Check sheet for the modelled part. Datum: model origin and axes. Units: mm. A direction names the side the tool comes from. Give positions to 0.01 mm unless a question says otherwise; leave off trailing zeros. Order: outer loops, then holes, each group sorted by start corner. A loop starts at its lowest first (then second) coordinate and runs counter-clockwise, first axis right, second up. Notation, with made-up numbers: (78, 17.25) - (103, 17.25) arc R26 cw to (103, 48.25) - close; hole circle Ø1 at (14, 34.25). An arc over 180 degrees is marked (long way). Answer in a Markdown table with one row per item.
from build123d import *

# Parameters (mm, degrees)
SKETCH1_R           = 11
BOSS_EXTRUDE1_DEPTH = 1.5
SKETCH4_R           = 12.5
BOSS_EXTRUDE2_DEPTH = 3
SKETCH5_R           = 1.45
CUT_EXTRUDE1_DEPTH  = 2
SKETCH6_R           = 1.5
CUT_EXTRUDE2_DEPTH  = 2


with BuildPart() as part:
    # Sketch1 → Boss-Extrude1 (new, symmetric)
    with BuildSketch(Plane.XY):
        Circle(SKETCH1_R)
    extrude(amount=BOSS_EXTRUDE1_DEPTH, both=True)

    # Sketch2 → Revolve1 (revolve)
    with BuildSketch(Plane(origin=(0, 0, 0), x_dir=(0, 0, -1), z_dir=(1, 0, 0)), mode=Mode.PRIVATE) as revolve1_sk:
        Polygon((-4.5, 0), (-4.5, 12.5), (-1.5, 11.096489402), (-1.5, 0), align=None)
    revolve(revolve1_sk.sketch.rotate(Axis((0, 0, 0), (0, 0, 1)), 90), axis=Axis((0, 0, 0), (0, 0, 1)))

    # Sketch4 → Boss-Extrude2 (add)
    with BuildSketch(Plane.XY.offset(4.5)):
        Circle(SKETCH4_R)
    extrude(amount=BOSS_EXTRUDE2_DEPTH)

    # Sketch5 → Cut-Extrude1 (cut)
    with BuildSketch(Plane.XY.offset(7.5)):
        with Locations((0, 9.315)):
            Circle(SKETCH5_R)
        with Locations((9.315, 0)):
            Circle(SKETCH5_R)
        with Locations((0, -9.315)):
            Circle(SKETCH5_R)
        with Locations((-9.315, 0)):
            Circle(SKETCH5_R)
    extrude(amount=-CUT_EXTRUDE1_DEPTH, mode=Mode.SUBTRACT)

    # Sketch6 → Cut-Extrude2 (cut)
    with BuildSketch(Plane(origin=(0, 0, -1.5), x_dir=(-1, 0, 0), z_dir=(0, 0, -1))):
        with Locations((0, 7.5)):
            Circle(SKETCH6_R)
        with Locations((7.5, 0)):
            Circle(SKETCH6_R)
        with Locations((0, -7.5)):
            Circle(SKETCH6_R)
        with Locations((-7.5, 0)):
            Circle(SKETCH6_R)
    extrude(amount=-CUT_EXTRUDE2_DEPTH, mode=Mode.SUBTRACT)


solid = part.part
(1) Cross-section at A-A, the plane x = 0. Record the cut outline in (y, z) (3 decimals), then the cut area to 3 significant figures.
Geometry says:
| item | result |
|---|---|
| outline | (-12.5, 4.5) - (-11.096, 1.5) - (-11, 1.5) - (-11, -1.5) - (-9, -1.5) - (-9, 0.5) - (-6, 0.5) - (-6, -1.5) - (6, -1.5) - (6, 0.5) - (9, 0.5) - (9, -1.5) - (11, -1.5) - (11, 1.5) - (11.096, 1.5) - (12.5, 4.5) - (12.5, 7.5) - (10.765, 7.5) - (10.765, 5.5) - (7.865, 5.5) - (7.865, 7.5) - (-7.865, 7.5) - (-7.865, 5.5) - (-10.765, 5.5) - (-10.765, 7.5) - (-12.5, 7.5) - close |
| area | 188 mm² |
(2) Mould release check, pull along X, two halves, no side actions. Record for faces 1 (the flat face through (-9, 0, 5.5)), 2 (the cylindrical face through (11.923, 3.755, 5.979)), 3 (the flat face through (0, 0, -1.5)): pulls with the +X half, pulls with the -X half, needs draft (parallel to the pull), parting line crosses it, or undercut.
Geometry says:
| item | result |
|---|---|
| face 1 | undercut |
| face 2 | parting line crosses it |
| face 3 | needs draft |
(3) Thickness scan on L1, parallel to Y at x = 0, z = -0.25; L2, parallel to Y at x = 0, z = 5.9 (3 decimals); L3, parallel to Y at x = -10, z = 6.75. Record the ranges inside material, lowest first.
Geometry says:
| item | result |
|---|---|
| L1 | -11 to -9, -6 to 6, 9 to 11 |
| L2 | -12.5 to -10.765, -7.865 to 7.865, 10.765 to 12.5 |
| L3 | -7.5 to -1.28, 1.28 to 7.5 |
(4) Cross-section at B-B, the plane z = 3. Record the cut outline in (x, y), then the cut area to 3 significant figures.
Geometry says:
| item | result |
|---|---|
| outline | circle Ø23.6 at (0, 0) |
| area | 437 mm² |
(5) Gauge pin test, flat ends, axial feed: P1, Ø1, axis at x = -3, z = 2, coming from the +Y side; P2, Ø3.5, axis at x = 7.5, y = 0, coming from the -Z side; P3, Ø0.9, axis at x = 8.5, y = -0.5, coming from the +Z side; P4, Ø2, axis at y = 3.5, z = 5, coming from the +X side. Record the tip position at first contact, or that the pin passes through.
Geometry says:
| item | result |
|---|---|
| P1 | y = 11.2 |
| P2 | z = -1.5 |
| P3 | z = 5.5 |
| P4 | x = 12.25 |
(6) Access from +Z, -Z, +X, -X, +Y, -Y to the whole of each face (thin tool, end or side, straight path). Record for faces 4 (the cylindrical face through (10.698, 0.436, 6.514)), 5 (the cylindrical face through (-6, 0, -1)), 6 (the flat face through (0, 0, 7.5)).
Geometry says:
| item | result |
|---|---|
| face 4 | +Z |
| face 5 | -Z |
| face 6 | +Z, +X, -X, +Y, -Y |
